Can you work these out from the model? Positions are in its coordinate system, mm. Face numbers are marked on the shaded views. A direction names the side the tool comes from. Give positions to 0.01 mm unless a question says otherwise; leave off trailing zeros. Loops run counter-clockwise (first coordinate to the right, second up) from the corner with the lowest first, then second, coordinate; pieces in that order, holes last. Notation, with made-up numbers: (-10.75, 65.25) -> (-5.75, 65.25) arc R23 cw to (-5.75, 78.25) -> close; hole circle Ø4 at (45, -24.5). An arc over 180 degrees is marked (long way). Return JSON: item names as keys, results as strings. Group by question number.
Q1. Suppose I cut it at A-A, the plane y = 15. Please give me the cut outline in (x, z) (3 decimals), and give its area (3 significant figures).
Q2. I need wall thicknesses on line 1 along Z through (x, y) = (0, 6) (3 decimals); line 2 along Y through (x, z) = (1.5, 4.25); line 3 along Z through (x, y) = (2.5, 30). Which ranges of each line are inside material? Lowest first, please. Write a range as [from, to].
Q3. Will these pins go through, and if not, where does the flat tip stop? pin 1 (3 mm diameter, centred on y = 23.5, z = -2.5, fed in from +X); pin 2 (6 mm diameter, centred on y = 17.5, z = 1, fed in from -X) (3 decimals); pin 3 (2 mm diameter, centred on x = -0.5, y = 30, fed in from +Z) (3 decimals).
Q4. Which directions (+Z, -Z, +X, -X, +Y, -Y) give clear straight access to the entire face, cutting with the end or side of a thin tool? Please do the marked faces 1 and 2.
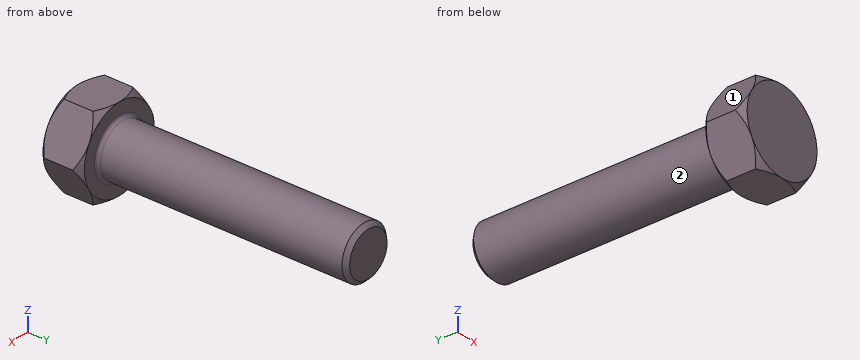
Autodesk Inventor part; units mm, degrees
ref_plane "YZ Plane" through (0, 0, 0) normal (1, 0, 0) x (0, 1, 0)
ref_plane "XZ Plane" through (0, 0, 0) normal (0, 1, 0) x (-1, 0, 0)
ref_plane "XY Plane" through (0, 0, 0) normal (0, 0, 1) x (1, 0, 0)
sketch "Esboço1" plane through (0, 0, 0) normal (0, 1, 0) x (-1, 0, 0)
  circle A0 centre (0, 0) radius 3
  line L0 (-2.8868, -5) -> (-5.7735, 0)
  line L1 (-5.7735, 0) -> (-2.8868, 5)
  line L2 (-2.8868, 5) -> (2.8868, 5)
  line L3 (2.8868, 5) -> (5.7735, 0)
  line L4 (5.7735, 0) -> (2.8868, -5)
  line L5 (2.8868, -5) -> (-2.8868, -5)
  dimension "d0" = 6
extrude "Extrusão1" add sketch "Esboço1" along normal blind 5
sketch "Esboço2" plane through (0, 0, 0) normal (1, 0, 0) x (0, 1, 0)
  point P0 (0, 0)
chamfer "Chanfro1" distance 0.5 angle 45 2 edges at (3, 0, 0) (3, 5, 0)
sketch "Esboço5" plane through (0, 0, 0) normal (0, -1, 0) x (1, 0, 0)
  circle A0 centre (0, 0) radius 5
extrude "Extrusão2" cut sketch "Esboço5" against normal through all draft 45 keep common part
sketch "Esboço6" plane through (0, 5, 0) normal (0, 1, 0) x (1, 0, 0)
  circle A0 centre (0, 0) radius 5
extrude "Extrusão3" cut sketch "Esboço6" against normal through all draft 45 keep common part
sketch "Esboço7" plane through (0, 5, 0) normal (0, 1, 0) x (1, 0, 0)
  circle A0 centre (0, 0) radius 3.5
extrude "Extrusão4" add sketch "Esboço7" against normal blind 5
sketch "Esboço8" plane through (0, 5, 0) normal (0, 1, 0) x (1, 0, 0)
  circle A0 centre (0, 0) radius 3.175
  dimension "d16" = 6.35
extrude "Extrusão5" add sketch "Esboço8" along normal blind 30
fillet "Arredondamento2" radius 0.4 1 edges at (-3.175, 5, 0)
chamfer "Chanfro3" distance 0.5 angle 45 1 edges at (-3.175, 35, 0)
thread "Rosca3"
properties part number "Parafuso sextavado 1 quarto 30mm" material "Aço inoxidável"
Ans:
{
 "1": {"outline": "circle Ø6.35 at (0, 0)", "area": "31.7 mm^2"},
 "2": {"line 1": "z = [-3.175, 3.175]", "line 2": "y = [0, 5]", "line 3": "z = [-1.96, 1.96]"},
 "3": {"pin 1": "stops at x = 3.01", "pin 2": "stops at x = -3.175", "pin 3": "stops at z = 3.175"},
 "4": {"face 1": "+Z, -X, +Y, -Y", "face 2": "+Y"}
}
